Build history of the part. All positions in model axes, mm. Round coordinates to 2 decimals unless told otherwise and drop trailing zeros. Write each loop counter-clockwise with the first axis right and the second up, starting at its lowest first coordinate (ties: lowest second). Pieces come first, ordered by that corner, then holes. Notation, with made-up numbers: (32.25, 9) - (78.25, 9) arc R16 ccw to (78.25, 27) - close; hole circle Ø7 at (4.25, 15). An arc over 180 degrees is marked (long way). Write each question's results on one line, items separated by ' | '.
from build123d import *

# Parameters (mm, degrees)
SKETCH_1_R          = 250
EXTRUDE_1_DEPTH     = 5
SKETCH_2_R          = 2.5
CUT_EXTRUDE_1_DEPTH = 354.588744165
SKETCH_3_R          = 2.5
CUT_EXTRUDE_2_DEPTH = 354.588744165
CUT_EXTRUDE4_DEPTH  = 354.588744165


with BuildPart() as part:
    # Sketch 1 → Extrude 1 (new body)
    with BuildSketch(Plane(origin=(0, 0, 0), x_dir=(1, 0, 0), z_dir=(0, 1, 0))):
        with Locations(Location((0, 0, 0), (0, 0, 270))):
            Circle(SKETCH_1_R)
    extrude(amount=EXTRUDE_1_DEPTH)

    # Sketch 2 → Cut-Extrude 1 (cut, through all)
    with BuildSketch(Plane(origin=(0, 5, 0), x_dir=(1, 0, 0), z_dir=(0, 1, 0))):
        with Locations(Location((-220, -29, 0), (0, 0, 270))):
            Circle(SKETCH_2_R)
        with Locations(Location((-220, 29, 0), (0, 0, 270))):
            Circle(SKETCH_2_R)
        with Locations(Location((-175, -29, 0), (0, 0, 270))):
            Circle(SKETCH_2_R)
        with Locations(Location((-175, 29, 0), (0, 0, 270))):
            Circle(SKETCH_2_R)
        with Locations(Location((84.88526329, 205.025588833, 0), (0, 0, 270))):
            Circle(SKETCH_2_R)
        with Locations(Location((135.11473671, 176.025588833, 0), (0, 0, 270))):
            Circle(SKETCH_2_R)
        with Locations(Location((62.38526329, 166.054445662, 0), (0, 0, 270))):
            Circle(SKETCH_2_R)
        with Locations(Location((112.61473671, 137.054445662, 0), (0, 0, 270))):
            Circle(SKETCH_2_R)
        with Locations(Location((135.11473671, -176.025588833, 0), (0, 0, 270))):
            Circle(SKETCH_2_R)
        with Locations(Location((84.88526329, -205.025588833, 0), (0, 0, 270))):
            Circle(SKETCH_2_R)
        with Locations(Location((112.61473671, -137.054445662, 0), (0, 0, 270))):
            Circle(SKETCH_2_R)
        with Locations(Location((62.38526329, -166.054445662, 0), (0, 0, 270))):
            Circle(SKETCH_2_R)
    extrude(amount=-CUT_EXTRUDE_1_DEPTH, mode=Mode.SUBTRACT)

    # Sketch 3 → Cut-Extrude 2 (cut, through all)
    with BuildSketch(Plane(origin=(0, 5, 0), x_dir=(1, 0, 0), z_dir=(0, 1, 0))):
        with Locations(Location((163, 135, 0), (0, 0, 90))):
            Circle(SKETCH_3_R)
        with Locations(Location((105, 135, 0), (0, 0, 90))):
            Circle(SKETCH_3_R)
        with Locations(Location((105, 180, 0), (0, 0, 90))):
            Circle(SKETCH_3_R)
        with Locations(Location((163, 180, 0), (0, 0, 90))):
            Circle(SKETCH_3_R)
        with Locations(Location((-163, 180, 0), (0, 0, 270))):
            Circle(SKETCH_3_R)
        with Locations(Location((-105, 180, 0), (0, 0, 270))):
            Circle(SKETCH_3_R)
        with Locations(Location((-105, 135, 0), (0, 0, 270))):
            Circle(SKETCH_3_R)
        with Locations(Location((-163, 135, 0), (0, 0, 270))):
            Circle(SKETCH_3_R)
        with Locations(Location((-163, -135, 0), (0, 0, 90))):
            Circle(SKETCH_3_R)
        with Locations(Location((-105, -135, 0), (0, 0, 90))):
            Circle(SKETCH_3_R)
        with Locations(Location((-105, -180, 0), (0, 0, 90))):
            Circle(SKETCH_3_R)
        with Locations(Location((-163, -180, 0), (0, 0, 90))):
            Circle(SKETCH_3_R)
        with Locations(Location((163, -180, 0), (0, 0, 270))):
            Circle(SKETCH_3_R)
        with Locations(Location((105, -180, 0), (0, 0, 270))):
            Circle(SKETCH_3_R)
        with Locations(Location((105, -135, 0), (0, 0, 270))):
            Circle(SKETCH_3_R)
        with Locations(Location((163, -135, 0), (0, 0, 270))):
            Circle(SKETCH_3_R)
        with Locations(Location((-62.5, 62.5, 0), (0, 0, 270))):
            Circle(SKETCH_3_R)
        with Locations(Location((62.5, 62.5, 0), (0, 0, 90))):
            Circle(SKETCH_3_R)
        with Locations(Location((62.5, -62.5, 0), (0, 0, 270))):
            Circle(SKETCH_3_R)
        with Locations(Location((-62.5, -62.5, 0), (0, 0, 90))):
            Circle(SKETCH_3_R)
    extrude(amount=-CUT_EXTRUDE_2_DEPTH, mode=Mode.SUBTRACT)

    # Sketch2 → Cut-Extrude4 (cut, through all)
    with BuildSketch(Plane.XZ):
        with BuildLine():
            Line((-50, 40), (-50, -40))
            ThreePointArc((-50, -40), (-47.071067812, -47.071067812), (-40, -50))
            Line((-40, -50), (40, -50))
            ThreePointArc((40, -50), (47.071067812, -47.071067812), (50, -40))
            Line((50, -40), (50, 40))
            ThreePointArc((50, 40), (47.071067812, 47.071067812), (40, 50))
            Line((40, 50), (-40, 50))
            ThreePointArc((-40, 50), (-47.071067812, 47.071067812), (-50, 40))
        make_face()
    extrude(amount=-CUT_EXTRUDE4_DEPTH, mode=Mode.SUBTRACT)


solid = part.part
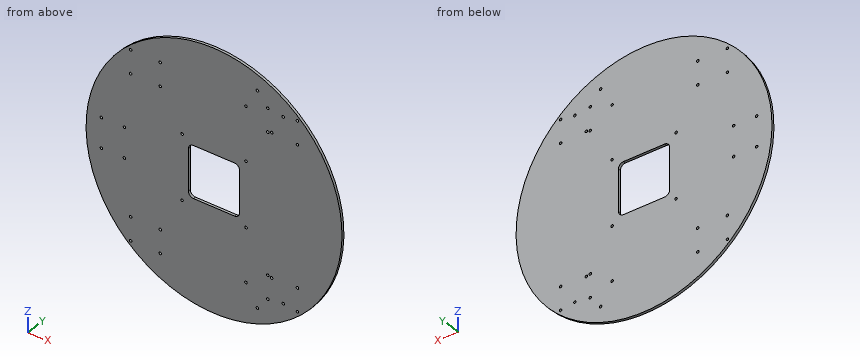
(1) Slice it at A-A, the plane z = 0. Write the cut outline in (x, y).
Worked answers:
outline: (-250, 0) - (-50, 0) - (-50, 5) - (-250, 5) - close; (50, 0) - (250, 0) - (250, 5) - (50, 5) - close
(2) Flat gauge pins, fed straight in: pin 1 Ø4 at (x, z) = (-163, 135) entering from -Y; pin 2 Ø1 at (x, y) = (-82.5, 3) entering from +Z; pin 3 Ø3 at (x, y) = (-116.5, 3) entering from +Z; pin 4 Ø2 at (y, z) = (2, 27.5) entering from -X. Where does each tip first touch, or does it go through?
Worked answers:
pin 1: passes through | pin 2: stops at z = 236.17 | pin 3: stops at z = 221.98 | pin 4: stops at x = -248.59
(3) Slice it at D-D, the plane x = 210. Write the cut outline in (y, z), and give its area (3 significant figures).
Worked answers:
outline: (0, -135.65) - (5, -135.65) - (5, 135.65) - (0, 135.65) - close | area: 1,360 mm2
(4) Slice it at B-B, the plane x = 0. Write the cut outline in (y, z).
Worked answers:
outline: (0, -250) - (5, -250) - (5, -50) - (0, -50) - close; (0, 50) - (5, 50) - (5, 250) - (0, 250) - close
(5) Slice it at C-C, the plane y = 4.2. State how many separate pieces and enclosed holes the cut face has, and give its area (3 significant figures).
Worked answers:
separate pieces: 1 | enclosed holes: 33 | area: 186,000 mm2
(6) Drill centre lines: probe 1 along X at (y, z) = (1.85, -180); probe 2 along Z at (x, y) = (164, 1.3); probe 3 along X at (y, z) = (2.8, 29). Where is each one in solid material? Low to high. Write a range as [from, to].
Worked answers:
probe 1: x = [-173.49, -165.5], [-160.5, -107.5], [-102.5, 102.5], [107.5, 160.5], [165.5, 173.49] | probe 2: z = [-188.69, -182.29], [-177.71, -137.29], [-132.71, 132.71], [137.29, 177.71], [182.29, 188.69] | probe 3: x = [-248.31, -222.5], [-217.5, -177.5], [-172.5, -50], [50, 248.31]
